For this review, take the finished solid that the model builds, in its own axes (mm). Face numbers are marked on the shaded views. A direction names the side the tool comes from. Give positions to 0.01 mm unless a question says otherwise; leave off trailing zeros. Order: outer loops, then holes, each group sorted by start corner. A loop starts at its lowest first (then second) coordinate and runs counter-clockwise, first axis right, second up. Notation, with made-up numbers: (-30.75, -12.75) -> (8.25, -12.75) arc R17 cw to (8.25, 5.25) -> close; hole circle Ø9 at (48, -38). An arc over 180 degrees is marked (long way). Return JSON: item names as keys, results as strings. Group by question number.
1) Add section A-A (z = 19.5). Give the boundary of the cut face in (x, y).
2) To check wall thickness, follow line 1 along X through (y, z) = (-13.5, 9.5); line 2 along Y through (x, z) = (106.5, 12.75); line 3 along X through (y, z) = (-90.5, 19.5). State the ranges of each line that lie inside material, in increasing order.
3) Add section B-B (y = -30). Give the boundary of the cut face in (x, z).
4) The part is to be moulded in two halves that separate along Y. For the marked faces 3, 4 and 5, say which applies: released by +Y, released by -Y, zero draft, split by the parting line, or undercut.
5) For the marked faces 1 and 2, list the 3-axis set-ups (+Z, -Z, +X, -X, +Y, -Y) from which the entire face can be reached by the end or side of a thin tool; tool diameter is ignored.
6) Add section C-C (x = 84). Give the boundary of the cut face in (y, z), then the cut area to 3 significant figures.
from build123d import *

# Parameters (mm, degrees)
F1_DEPTH = 25
F2_DEPTH = 3
F3_R     = 2
F4_R     = 2
F5_SIZE  = 1


with BuildPart() as f1:
    # F0 (on Top) → F1 (new body)
    with BuildSketch(Plane.XY):
        with BuildLine():
            Line((180.736435, 0), (0.736435, 0))
            ThreePointArc((0.736435, 0), (-6.334633, -2.928932), (-9.263565, -10))
            Line((-9.263565, -10), (-9.263565, -90))
            ThreePointArc((-9.263565, -90), (-6.334633, -97.071068), (0.736435, -100))
            Line((0.736435, -100), (180.736435, -100))
            ThreePointArc((180.736435, -100), (187.807502, -97.071068), (190.736435, -90))
            Line((190.736435, -90), (190.736435, -10))
            ThreePointArc((190.736435, -10), (187.807502, -2.928932), (180.736435, 0))
        make_face()
        with BuildLine():
            ThreePointArc((-6.263565, -10), (-4.213313, -5.050253), (0.736435, -3))
            Line((0.736435, -3), (180.736435, -3))
            ThreePointArc((180.736435, -3), (185.686182, -5.050253), (187.736435, -10))
            Line((187.736435, -10), (187.736435, -90))
            ThreePointArc((187.736435, -90), (185.686182, -94.949747), (180.736435, -97))
            Line((180.736435, -97), (0.736435, -97))
            ThreePointArc((0.736435, -97), (-4.213313, -94.949747), (-6.263565, -90))
            Line((-6.263565, -90), (-6.263565, -10))
        make_face(mode=Mode.SUBTRACT)
    extrude(amount=F1_DEPTH)

    # F0 (on Top) → F2 (join)
    with BuildSketch(Plane.XY):
        with BuildLine():
            Line((180.736435, -3), (0.736435, -3))
            ThreePointArc((0.736435, -3), (-4.213313, -5.050253), (-6.263565, -10))
            Line((-6.263565, -10), (-6.263565, -90))
            ThreePointArc((-6.263565, -90), (-4.213313, -94.949747), (0.736435, -97))
            Line((0.736435, -97), (180.736435, -97))
            ThreePointArc((180.736435, -97), (185.686182, -94.949747), (187.736435, -90))
            Line((187.736435, -90), (187.736435, -10))
            ThreePointArc((187.736435, -10), (185.686182, -5.050253), (180.736435, -3))
        make_face()
    extrude(amount=F2_DEPTH)

    # F3
    f3_edges = [f1.edges().sort_by_distance(p)[0] for p in [
        (-6.263565, -50, 3),
        (-4.213313, -5.050253, 3),
        (90.736435, -3, 3),
        (-4.213313, -94.949747, 3),
        (90.736435, -97, 3),
        (185.686182, -94.949747, 3),
        (187.736435, -50, 3),
        (185.686182, -5.050253, 3),
    ]]
    fillet(f3_edges, radius=F3_R)

    # F4
    f4_edges = [f1.edges().sort_by_distance(p)[0] for p in [
        (90.736435, -100, 0),
        (187.807502, -2.928932, 0),
        (90.736435, 0, 0),
        (-6.334633, -2.928932, 0),
        (-9.263565, -50, 0),
        (-6.334633, -97.071068, 0),
        (187.807502, -97.071068, 0),
        (190.736435, -50, 0),
    ]]
    fillet(f4_edges, radius=F4_R)

    # F5
    f5_edges = [f1.edges().sort_by_distance(p)[0] for p in [
        (-9.263565, -50, 25),
        (-6.334633, -97.071068, 25),
        (90.736435, -100, 25),
        (187.807502, -97.071068, 25),
        (190.736435, -50, 25),
        (187.807502, -2.928932, 25),
        (90.736435, 0, 25),
    ]]
    chamfer(f5_edges, length=F5_SIZE)


solid = f1.part
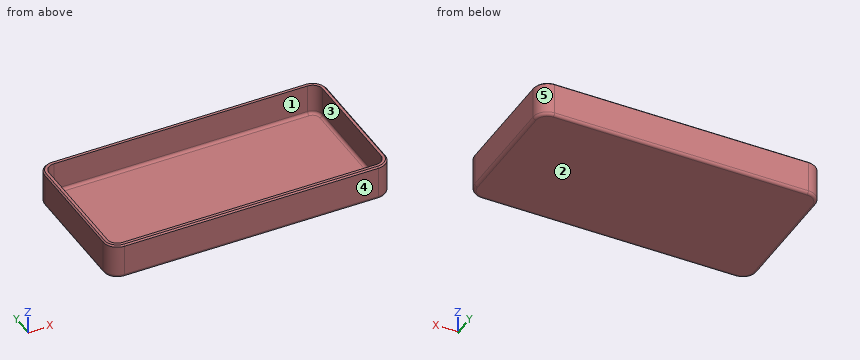
Evaluation:
{
 "1": {"outline": "(-9.26, -90) arc R10 ccw to (0.74, -100) -> (180.74, -100) arc R10 ccw to (190.74, -90) -> (190.74, -10) arc R10 ccw to (180.74, 0) -> (0.74, 0) arc R10 ccw to (-9.26, -10) -> close; hole (-6.26, -90) arc R7 ccw to (0.74, -97) -> (180.74, -97) arc R7 ccw to (187.74, -90) -> (187.74, -10) arc R7 ccw to (180.74, -3) -> (0.74, -3) arc R7 ccw to (-6.26, -10) -> close"},
 "2": {"line 1": "-9.26 to -6.26, 187.74 to 190.74", "line 2": "-100 to -97, -3 to 0", "line 3": "-9.25 to -6.25, 187.72 to 190.72"},
 "3": {"outline": "(-9.26, 2) arc R2 ccw to (-7.26, 0) -> (188.74, 0) arc R2 ccw to (190.74, 2) -> (190.74, 24) -> (189.74, 25) -> (187.74, 25) -> (187.74, 5) arc R2 cw to (185.74, 3) -> (-4.26, 3) arc R2 cw to (-6.26, 5) -> (-6.26, 25) -> (-8.26, 25) -> (-9.26, 24) -> close"},
 "4": {"face 3": "undercut", "face 4": "released by -Y", "face 5": "released by +Y"},
 "5": {"face 1": "+Z", "face 2": "-Z, +X, -X, +Y, -Y"},
 "6": {"outline": "(-100, 2) arc R2 ccw to (-98, 0) -> (-2, 0) arc R2 ccw to (0, 2) -> (0, 24) -> (-1, 25) -> (-3, 25) -> (-3, 5) arc R2 cw to (-5, 3) -> (-95, 3) arc R2 cw to (-97, 5) -> (-97, 25) -> (-99, 25) -> (-100, 24) -> close", "area": "431 mm^2"}
}
